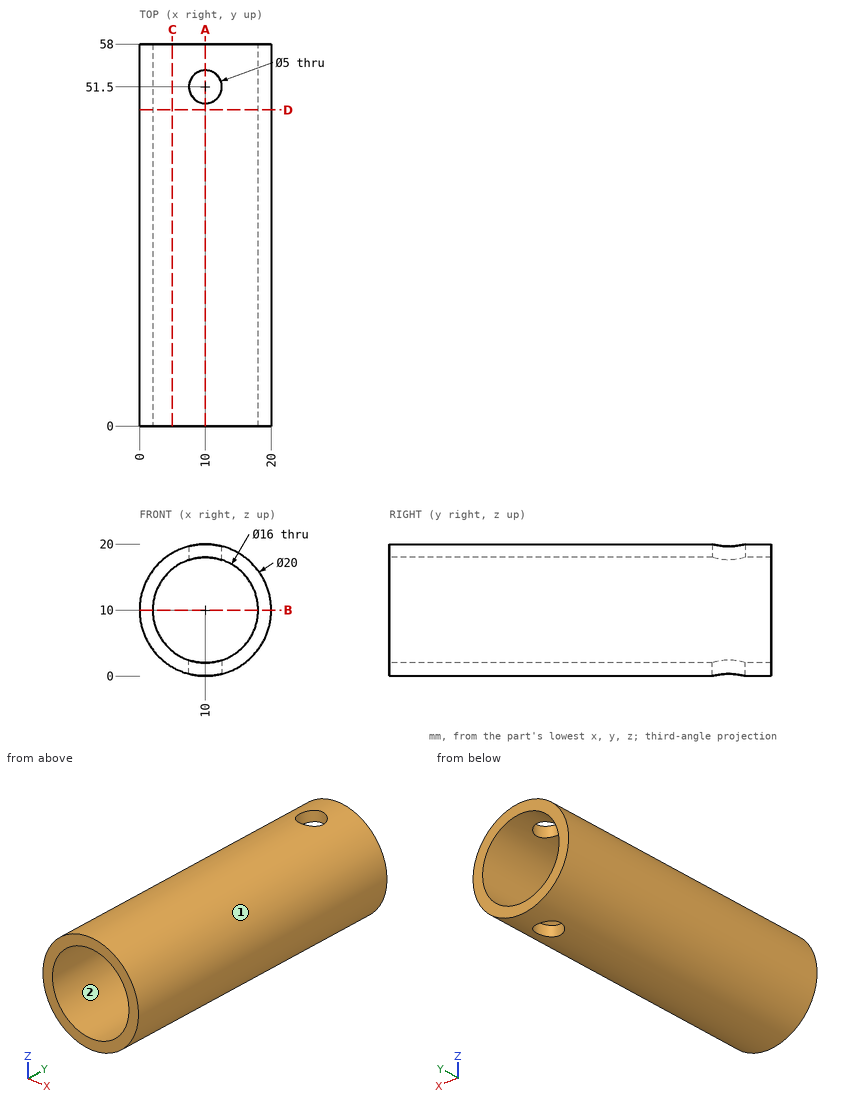
Geometry check sheet. Reference: drawing and pictorial views, mm from the part's lowest x, y, z. Round coordinates to 2 decimals unless told otherwise and drop trailing zeros. Order: outer loops, then holes, each group sorted by start corner. A loop starts at its lowest first (then second) coordinate and runs counter-clockwise, first axis right, second up.
Q1. Scan lines: L1, parallel to Y at x = 10, z = 1.3; L2, parallel to Z at x = 5.5, y = 49.5; L3, parallel to Z at x = 16.75, y = 27. Record each from-to range of solid material in increasing order.
Filled sheet:
L1: y = 0 to 49, 54 to 58
L2: z = 1.07 to 3.39, 16.61 to 18.93
L3: z = 2.62 to 5.71, 14.29 to 17.38
Q2. Draft check along Z on the marked faces 1 and 2. Enter one of: pulls with the +Z half, pulls with the -Z half, needs draft (parallel to the pull), parting line crosses it, or undercut.
Filled sheet:
face 1: parting line crosses it
face 2: undercut
Q3. Cross-section at A-A, the plane x = 10. Enter the section's corners in (y, z).
Filled sheet:
outline: (0, 0) - (49, 0) - (49, 2) - (0, 2) - close; (0, 18) - (49, 18) - (49, 20) - (0, 20) - close; (54, 0) - (58, 0) - (58, 2) - (54, 2) - close; (54, 18) - (58, 18) - (58, 20) - (54, 20) - close
Q4. Cross-section at B-B, the plane z = 10. Enter the section's corners in (x, y).
Filled sheet:
outline: (0, 0) - (2, 0) - (2, 58) - (0, 58) - close; (18, 0) - (20, 0) - (20, 58) - (18, 58) - close
Q5. Depth check by flat-ended pin: P1, Ø1.5, axis at y = 20.5, z = 18, coming from the -X side; P2, Ø5, axis at x = 5.5, y = 21.5, coming from the -Z side; P3, Ø10, axis at x = 3.5, y = 7, coming from the +Z side. Enter the tip coordinate at first touch or a pass-through.
Filled sheet:
P1: stops at x = 3.11
P2: stops at z = 0.2
P3: stops at z = 19.89
Q6. Cross-section at C-C, the plane x = 5. Enter the section's corners in (y, z) (3 decimals).
Filled sheet:
outline: (0, 1.34) - (58, 1.34) - (58, 3.755) - (0, 3.755) - close; (0, 16.245) - (58, 16.245) - (58, 18.66) - (0, 18.66) - close
Q7. Cross-section at D-D, the plane y = 48. Enter the section's corners in (x, z), plus the area to 3 significant figures.
Filled sheet:
outline: circle Ø20 at (10, 10); hole circle Ø16 at (10, 10)
area: 113 mm2
